The model under review builds one solid part; all positions refer to its coordinate system, in mm. Give positions to 0.01 mm unless a question says otherwise; leave off trailing zeros. Loops run counter-clockwise (first coordinate to the right, second up) from the corner with the lowest first, then second, coordinate; pieces in that order, holes last. Notation, with made-up numbers: (-2, -6) - (52, -6) arc R30 cw to (52, 21) - close; hole circle Ø3 at (2.5, 81.5). An arc over 180 degrees is marked (long way). Return JSON: item names as keys, results as strings. Group by question number.
```python
from build123d import *

# Parameters (mm, degrees)
F0_R     = 25.975
F1_DEPTH = 2.5
F3_DEPTH = 3


with BuildPart() as f1:
    # F0 (on Top) → F1 (new body)
    with BuildSketch(Plane.XY):
        Circle(F0_R)
        Polygon((-13.86, 8.002075), (0, 16.004149), (13.86, 8.002075), (13.86, -8.002075), (0, -16.004149), (-13.86, -8.002075), align=None, mode=Mode.SUBTRACT)
    extrude(amount=F1_DEPTH)

    # F2 (on face) → F3 (cut)
    with BuildSketch(Plane.XY.offset(2.5)):
        with BuildLine():
            ThreePointArc((16.363608, 12.021167), (17.062582, 11.914235), (17.169515, 12.613209))
            ThreePointArc((17.169515, 12.613209), (15.766582, 14.3283), (14.1931, 15.888398))
            ThreePointArc((14.1931, 15.888398), (13.487113, 15.848611), (13.5269, 15.142625))
            ThreePointArc((13.5269, 15.142625), (15.026526, 13.655754), (16.363608, 12.021167))
        make_face()
        with BuildLine():
            ThreePointArc((8.160716, 18.59244), (8.819512, 18.849321), (8.562631, 19.508117))
            ThreePointArc((8.562631, 19.508117), (6.490111, 20.291962), (4.347386, 20.856306))
            ThreePointArc((4.347386, 20.856306), (3.755877, 20.468856), (4.143327, 19.877348))
            ThreePointArc((4.143327, 19.877348), (6.185476, 19.339493), (8.160716, 18.59244))
        make_face()
        with BuildLine():
            ThreePointArc((-2.228832, 20.181883), (-1.786739, 20.733747), (-2.338602, 21.17584))
            ThreePointArc((-2.338602, 21.17584), (-4.52538, 20.81841), (-6.663207, 20.235784))
            ThreePointArc((-6.663207, 20.235784), (-6.981743, 19.604488), (-6.350447, 19.285952))
            ThreePointArc((-6.350447, 19.285952), (-4.312967, 19.841231), (-2.228832, 20.181883))
        make_face()
        with BuildLine():
            ThreePointArc((-12.021167, 16.363608), (-11.914235, 17.062582), (-12.613209, 17.169515))
            ThreePointArc((-12.613209, 17.169515), (-14.3283, 15.766582), (-15.888398, 14.1931))
            ThreePointArc((-15.888398, 14.1931), (-15.848611, 13.487113), (-15.142625, 13.5269))
            ThreePointArc((-15.142625, 13.5269), (-13.655754, 15.026526), (-12.021167, 16.363608))
        make_face()
        with BuildLine():
            ThreePointArc((-18.59244, 8.160716), (-18.849321, 8.819512), (-19.508117, 8.562631))
            ThreePointArc((-19.508117, 8.562631), (-20.291962, 6.490111), (-20.856306, 4.347386))
            ThreePointArc((-20.856306, 4.347386), (-20.468856, 3.755877), (-19.877348, 4.143327))
            ThreePointArc((-19.877348, 4.143327), (-19.339493, 6.185476), (-18.59244, 8.160716))
        make_face()
        with BuildLine():
            ThreePointArc((-20.181883, -2.228832), (-20.733747, -1.786739), (-21.17584, -2.338602))
            ThreePointArc((-21.17584, -2.338602), (-20.81841, -4.52538), (-20.235784, -6.663207))
            ThreePointArc((-20.235784, -6.663207), (-19.604488, -6.981743), (-19.285952, -6.350447))
            ThreePointArc((-19.285952, -6.350447), (-19.841231, -4.312967), (-20.181883, -2.228832))
        make_face()
        with BuildLine():
            ThreePointArc((-16.363608, -12.021167), (-17.062582, -11.914235), (-17.169515, -12.613209))
            ThreePointArc((-17.169515, -12.613209), (-15.766582, -14.3283), (-14.1931, -15.888398))
            ThreePointArc((-14.1931, -15.888398), (-13.487113, -15.848611), (-13.5269, -15.142625))
            ThreePointArc((-13.5269, -15.142625), (-15.026526, -13.655754), (-16.363608, -12.021167))
        make_face()
        with BuildLine():
            ThreePointArc((-8.160716, -18.59244), (-8.819512, -18.849321), (-8.562631, -19.508117))
            ThreePointArc((-8.562631, -19.508117), (-6.490111, -20.291962), (-4.347386, -20.856306))
            ThreePointArc((-4.347386, -20.856306), (-3.755877, -20.468856), (-4.143327, -19.877348))
            ThreePointArc((-4.143327, -19.877348), (-6.185476, -19.339493), (-8.160716, -18.59244))
        make_face()
        with BuildLine():
            ThreePointArc((2.228832, -20.181883), (1.786739, -20.733747), (2.338602, -21.17584))
            ThreePointArc((2.338602, -21.17584), (4.52538, -20.81841), (6.663207, -20.235784))
            ThreePointArc((6.663207, -20.235784), (6.981743, -19.604488), (6.350447, -19.285952))
            ThreePointArc((6.350447, -19.285952), (4.312967, -19.841231), (2.228832, -20.181883))
        make_face()
        with BuildLine():
            ThreePointArc((12.021167, -16.363608), (11.914235, -17.062582), (12.613209, -17.169515))
            ThreePointArc((12.613209, -17.169515), (14.3283, -15.766582), (15.888398, -14.1931))
            ThreePointArc((15.888398, -14.1931), (15.848611, -13.487113), (15.142625, -13.5269))
            ThreePointArc((15.142625, -13.5269), (13.655754, -15.026526), (12.021167, -16.363608))
        make_face()
        with BuildLine():
            ThreePointArc((18.59244, -8.160716), (18.849321, -8.819512), (19.508117, -8.562631))
            ThreePointArc((19.508117, -8.562631), (20.291962, -6.490111), (20.856306, -4.347386))
            ThreePointArc((20.856306, -4.347386), (20.468856, -3.755877), (19.877348, -4.143327))
            ThreePointArc((19.877348, -4.143327), (19.339493, -6.185476), (18.59244, -8.160716))
        make_face()
        with BuildLine():
            ThreePointArc((20.181883, 2.228832), (20.733747, 1.786739), (21.17584, 2.338602))
            ThreePointArc((21.17584, 2.338602), (20.81841, 4.52538), (20.235784, 6.663207))
            ThreePointArc((20.235784, 6.663207), (19.604488, 6.981743), (19.285952, 6.350447))
            ThreePointArc((19.285952, 6.350447), (19.841231, 4.312967), (20.181883, 2.228832))
        make_face()
    extrude(amount=-F3_DEPTH, mode=Mode.SUBTRACT)


solid = f1.part
```
1) We need section A-A, the plane y = 0. Write out the cut boundary in (x, z) (3 decimals).
2) We need section C-C, the plane z = 1.5. Count the separate pieces of the cut face and the enclosed holes in it, plus the area to 3 significant figures.
3) To check wall thickness, follow line 1 (Y direction, x = 15, z = 2.3); line 2 (Y direction, x = -7.5, z = 0.2); line 3 (Y direction, x = -6, z = 1.7). State the ranges of each line that lie inside material, in increasing order.
4) Draft analysis for pull direction X (two halves, no side actions). For faces 1 (the face through (-3.381, 25.754, 1.232)), 2 (the face through (15.787, 14.305, 1.268)), 3 (the face through (11, -11, 0)), state which applies: +X half, -X half, draft (parallel to the pull), parting line (faces both ways), or undercut.
5) For pin 1 Ø1 at (x, z) = (-3.5, 1.5) entering from +Y; pin 2 Ø1.5 at (x, z) = (-1.5, 0.5) entering from +Y, all flat-tipped, find the tip position at first contact; note any pin that passes through.
6) We need section B-B, the plane x = -10.5. Write out the cut boundary in (y, z), plus the area to 3 significant figures.
Findings:
{
 "1": {"outline": "(-25.975, 0) - (-13.86, 0) - (-13.86, 2.5) - (-25.975, 2.5) - close; (13.86, 0) - (25.975, 0) - (25.975, 2.5) - (13.86, 2.5) - close"},
 "2": {"separate pieces": "1", "enclosed holes": "13", "area": "1,390 mm^2"},
 "3": {"line 1": "y = -21.21 to -15.13, -13.68 to 13.68, 15.13 to 21.21", "line 2": "y = -24.87 to -19.94, -18.87 to -11.67, 11.67 to 24.87", "line 3": "y = -25.27 to -20.44, -19.4 to -12.54, 12.54 to 19.4, 20.44 to 25.27"},
 "4": {"face 1": "parting line", "face 2": "undercut", "face 3": "draft"},
 "5": {"pin 1": "stops at y = 25.8", "pin 2": "stops at y = 25.96"},
 "6": {"outline": "(-23.76, 0) - (-9.94, 0) - (-9.94, 2.5) - (-23.76, 2.5) - close; (9.94, 0) - (23.76, 0) - (23.76, 2.5) - (9.94, 2.5) - close", "area": "69.1 mm^2"}
}
